Part model, mm, in its own coordinate system. A direction names the side the tool comes from. Coordinates: 2 decimals unless noted, no trailing zeros. Order: outer loops, then holes, each group sorted by start corner. A loop starts at its lowest first (then second) coordinate and runs counter-clockwise, first axis right, second up. Notation, with made-up numbers: (9.25, -35.5) - (52.25, -35.5) arc R15 cw to (52.25, -12.5) - close; hole circle Ø3 at (88.25, -39.5). An arc over 180 degrees is marked (long way). Use a Markdown table: item, result. Add a question column.
1) Saw through at B-B on x = 65. List the corners of the cut face in (y, z) (3 decimals), then the cut area to 3 significant figures.
2) Tool access for faces 5 (the face through (3, -9.525, 0)), 6 (the face through (3, -12.7, 0)): list every direction of +Z, -Z, +X, -X, +Y, -Y with a clear straight run to the whole face (end or side of a thin tool).
3) Saw through at A-A on z = 5.75. List the corners of the cut face in (x, y) (3 decimals), then the cut area to 3 significant figures.
4) Wall check: L1, parallel to Y at x = -116, z = -0.75 (3 decimals); L2, parallel to Z at x = 127, y = 10.2. Give the ranges that are in metal, low to high. Write a range as [from, to].
5) Two-plate mould, pull along Z, no slides. Class faces 1 (the face through (190.5, 0, -11)), 2 (the face through (3, 9.525, 0)), 3 (the face through (3, 0, -12.7)), 4 (the face through (3, 0, -9.525)): +Z half, -Z half, draft (parallel to the pull), parting line (faces both ways), or undercut.
```python
from build123d import *

# Parameters (mm, degrees)
SKETCH1_W             = 25.4
SKETCH1_H             = 25.4
SKETCH1_W_2           = 19.05
SKETCH1_H_2           = 19.05
BOSS_EXTRUDE1_DEPTH   = 190.5
SKETCH3_W             = 2.4892
SKETCH3_H             = 25.4
SKETCH3_AT_POINT_2_W  = 2.4892
SKETCH3_AT_POINT_2_H  = 25.4
LPATTERN1_START       = -12.7
LPATTERN1_OUTLINE_R   = 2.4892
LPATTERN1_DEPTH       = 25.4
LPATTERN1_2_OUTLINE_R = 2.4892
LPATTERN1_2_DEPTH     = 25.4


# Read off the part's stored shape, not the designer's step: LPattern1
with BuildPart() as part:
    # Sketch1 → Boss-Extrude1 (new, symmetric)
    with BuildSketch(Plane(origin=(0, 0, 0), x_dir=(0, 0, -1), z_dir=(1, 0, 0))):
        Rectangle(SKETCH1_W, SKETCH1_H)
        Rectangle(SKETCH1_W_2, SKETCH1_H_2, mode=Mode.SUBTRACT)
    extrude(amount=BOSS_EXTRUDE1_DEPTH, both=True)

    # Sketch3 → #9 (0.196) Diameter Hole1 (revolve, cut)
    with BuildSketch(Plane(origin=(177.8, 12.7, 0), x_dir=(0, 0, 1), z_dir=(1, 0, 0))):
        with Locations((1.2446, 12.7)):
            Rectangle(SKETCH3_W, SKETCH3_H)
    revolve(axis=Axis((177.8, 19.05, 0), (0, -1, 0)), mode=Mode.SUBTRACT)

    # Sketch3 at point 2 (carried to point 2, square into its face) → #9 (0.196) Diameter Hole1 at 2 (revolve, cut)
    with BuildSketch(Plane(origin=(177.8, 0, 12.7), x_dir=(0, -1, 0), z_dir=(1, 0, 0))):
        with Locations((1.2446, 12.7)):
            Rectangle(SKETCH3_AT_POINT_2_W, SKETCH3_AT_POINT_2_H)
    revolve(axis=Axis((177.8, 0, 19.05), (0, 0, -1)), mode=Mode.SUBTRACT)

    # LPattern1 outline → LPattern1 (cut)
    with BuildSketch(Plane.XY.offset(LPATTERN1_START)):
        with Locations((152.4, 0)):
            Circle(LPATTERN1_OUTLINE_R)
        with Locations((127, 0)):
            Circle(LPATTERN1_OUTLINE_R)
        with Locations((101.6, 0)):
            Circle(LPATTERN1_OUTLINE_R)
        with Locations((76.2, 0)):
            Circle(LPATTERN1_OUTLINE_R)
        with Locations((50.8, 0)):
            Circle(LPATTERN1_OUTLINE_R)
        with Locations((25.4, 0)):
            Circle(LPATTERN1_OUTLINE_R)
        Circle(LPATTERN1_OUTLINE_R)
        with Locations((-25.4, 0)):
            Circle(LPATTERN1_OUTLINE_R)
        with Locations((-50.8, 0)):
            Circle(LPATTERN1_OUTLINE_R)
        with Locations((-76.2, 0)):
            Circle(LPATTERN1_OUTLINE_R)
        with Locations((-101.6, 0)):
            Circle(LPATTERN1_OUTLINE_R)
        with Locations((-127, 0)):
            Circle(LPATTERN1_OUTLINE_R)
        with Locations((-152.4, 0)):
            Circle(LPATTERN1_OUTLINE_R)
        with Locations((-177.8, 0)):
            Circle(LPATTERN1_OUTLINE_R)
    extrude(amount=LPATTERN1_DEPTH, mode=Mode.SUBTRACT)

    # LPattern1 2 outline → LPattern1 2 (cut)
    with BuildSketch(Plane(origin=(0, 0, 0), x_dir=(1, 0, 0), z_dir=(0, 1, 0)).offset(LPATTERN1_START)):
        with Locations((152.4, 0)):
            Circle(LPATTERN1_2_OUTLINE_R)
        with Locations((127, 0)):
            Circle(LPATTERN1_2_OUTLINE_R)
        with Locations((101.6, 0)):
            Circle(LPATTERN1_2_OUTLINE_R)
        with Locations((76.2, 0)):
            Circle(LPATTERN1_2_OUTLINE_R)
        with Locations((50.8, 0)):
            Circle(LPATTERN1_2_OUTLINE_R)
        with Locations((25.4, 0)):
            Circle(LPATTERN1_2_OUTLINE_R)
        Circle(LPATTERN1_2_OUTLINE_R)
        with Locations((-25.4, 0)):
            Circle(LPATTERN1_2_OUTLINE_R)
        with Locations((-50.8, 0)):
            Circle(LPATTERN1_2_OUTLINE_R)
        with Locations((-76.2, 0)):
            Circle(LPATTERN1_2_OUTLINE_R)
        with Locations((-101.6, 0)):
            Circle(LPATTERN1_2_OUTLINE_R)
        with Locations((-127, 0)):
            Circle(LPATTERN1_2_OUTLINE_R)
        with Locations((-152.4, 0)):
            Circle(LPATTERN1_2_OUTLINE_R)
        with Locations((-177.8, 0)):
            Circle(LPATTERN1_2_OUTLINE_R)
    extrude(amount=LPATTERN1_2_DEPTH, mode=Mode.SUBTRACT)


solid = part.part
```
Results are:
| question | item | result |
|---|---|---|
| 1 | outline | (-12.7, -12.7) - (12.7, -12.7) - (12.7, 12.7) - (-12.7, 12.7) - close; hole (-9.525, -9.525) - (9.525, -9.525) - (9.525, 9.525) - (-9.525, 9.525) - close |
| 1 | area | 282 mm2 |
| 2 | face 5 | +X, -X |
| 2 | face 6 | +Z, -Z, +X, -X, -Y |
| 3 | outline | (-190.5, -12.7) - (190.5, -12.7) - (190.5, -9.525) - (-190.5, -9.525) - close; (-190.5, 9.525) - (190.5, 9.525) - (190.5, 12.7) - (-190.5, 12.7) - close |
| 3 | area | 2,420 mm2 |
| 4 | L1 | [-12.7, -9.525], [9.525, 12.7] |
| 4 | L2 | [-12.7, -2.49], [2.49, 12.7] |
| 5 | face 1 | draft |
| 5 | face 2 | undercut |
| 5 | face 3 | -Z half |
| 5 | face 4 | undercut |
